Geometry: final body of the model. Coordinates: model frame, mm. Give positions to 0.01 mm unless a question says otherwise; leave off trailing zeros. Write each loop counter-clockwise with the first axis right and the second up, starting at its lowest first coordinate (ties: lowest second). Pieces come first, ordered by that corner, then holes.
```python
from build123d import *

# Parameters (mm, degrees)
SKETCH1_W           = 431.8
SKETCH1_H           = 381
BOSS_EXTRUDE1_DEPTH = 3.175
SKETCH7_R           = 14.3129
SKETCH7_R_2         = 2.5527
AXLE_HOLES_DEPTH    = 288.946419712
SKETCH10_R          = 3.2385
CUT_EXTRUDE5_DEPTH  = 288.946419712
CUT_EXTRUDE4_START  = -3.175
CUT_EXTRUDE4_DEPTH  = 3.175


# Read off the part's stored shape, not the designer's step: Cut-Extrude4
with BuildPart() as part:
    # Sketch1 → Boss-Extrude1 (new body)
    with BuildSketch(Plane(origin=(0, 0, 0), x_dir=(1, 0, 0), z_dir=(0, 1, 0))):
        Rectangle(SKETCH1_W, SKETCH1_H)
    extrude(amount=BOSS_EXTRUDE1_DEPTH)

    # Sketch7 → Axle Holes (cut, through all)
    with BuildSketch(Plane(origin=(0, 3.175, 0), x_dir=(1, 0, 0), z_dir=(0, 1, 0))):
        with Locations(Location((124.4092, -152.4, 0), (0, 0, 270))):
            Circle(SKETCH7_R)
        with Locations(Location((124.4092, 152.4, 0), (0, 0, 270))):
            Circle(SKETCH7_R)
        with Locations(Location((25.4, 152.4, 0), (0, 0, 270))):
            Circle(SKETCH7_R)
        with Locations(Location((25.4, -152.4, 0), (0, 0, 270))):
            Circle(SKETCH7_R)
        with Locations(Location((0, 152.4, 0), (0, 0, 270))):
            Circle(SKETCH7_R_2)
        with Locations(Location((7.439487758, 170.360512242, 0), (0, 0, 270))):
            Circle(SKETCH7_R_2)
        with Locations(Location((25.4, 177.8, 0), (0, 0, 270))):
            Circle(SKETCH7_R_2)
        with Locations(Location((43.360512242, 170.360512242, 0), (0, 0, 270))):
            Circle(SKETCH7_R_2)
        with Locations(Location((25.4, -127, 0), (0, 0, 270))):
            Circle(SKETCH7_R_2)
        with Locations(Location((43.360512242, -134.439487758, 0), (0, 0, 270))):
            Circle(SKETCH7_R_2)
        with Locations(Location((50.8, -152.4, 0), (0, 0, 270))):
            Circle(SKETCH7_R_2)
        with Locations(Location((43.360512242, -170.360512242, 0), (0, 0, 270))):
            Circle(SKETCH7_R_2)
        with Locations(Location((50.8, 152.4, 0), (0, 0, 270))):
            Circle(SKETCH7_R_2)
        with Locations(Location((43.360512242, 134.439487758, 0), (0, 0, 270))):
            Circle(SKETCH7_R_2)
        with Locations(Location((25.4, 127, 0), (0, 0, 270))):
            Circle(SKETCH7_R_2)
        with Locations(Location((7.439487758, 134.439487758, 0), (0, 0, 270))):
            Circle(SKETCH7_R_2)
        with Locations(Location((25.4, -177.8, 0), (0, 0, 270))):
            Circle(SKETCH7_R_2)
        with Locations(Location((7.439487758, -170.360512242, 0), (0, 0, 270))):
            Circle(SKETCH7_R_2)
        with Locations(Location((0, -152.4, 0), (0, 0, 270))):
            Circle(SKETCH7_R_2)
        with Locations(Location((7.439487758, -134.439487758, 0), (0, 0, 270))):
            Circle(SKETCH7_R_2)
    extrude(amount=-AXLE_HOLES_DEPTH, mode=Mode.SUBTRACT)

    # Sketch10 → Cut-Extrude5 (cut, through all)
    with BuildSketch(Plane(origin=(0, 3.175, 0), x_dir=(1, 0, 0), z_dir=(0, 1, 0))):
        with Locations(Location((-9.525, -182.394929259, 0), (0, 0, 270))):
            Circle(SKETCH10_R)
        with Locations(Location((74.9046, -184.15, 0), (0, 0, 270))):
            Circle(SKETCH10_R)
        with Locations(Location((74.9046, -133.35, 0), (0, 0, 270))):
            Circle(SKETCH10_R)
        with Locations(Location((167.623037844, -168.275, 0), (0, 0, 270))):
            Circle(SKETCH10_R)
        with Locations(Location((167.623037844, 168.275, 0), (0, 0, 90))):
            Circle(SKETCH10_R)
        with Locations(Location((74.9046, 184.15, 0), (0, 0, 90))):
            Circle(SKETCH10_R)
        with Locations(Location((74.9046, 133.35, 0), (0, 0, 90))):
            Circle(SKETCH10_R)
        with Locations(Location((-9.525, 182.394929259, 0), (0, 0, 90))):
            Circle(SKETCH10_R)
    extrude(amount=-CUT_EXTRUDE5_DEPTH, mode=Mode.SUBTRACT)

    # Cut-Extrude4 outline → Cut-Extrude4 (cut)
    with BuildSketch(Plane(origin=(0, 3.175, 0), x_dir=(1, 0, 0), z_dir=(0, 1, 0)).offset(CUT_EXTRUDE4_START)):
        with BuildLine():
            Line((170.541801783, -180.70028669), (133.121928175, -189.490408029))
            ThreePointArc((133.121928175, -189.490408029), (128.794713317, -190.246760402), (124.4092, -190.5))
            Line((124.4092, -190.5), (215.9, -190.5))
            Line((215.9, -190.5), (215.9, 190.5))
            Line((215.9, 190.5), (124.4092, 190.5))
            ThreePointArc((124.4092, 190.5), (128.794713317, 190.246760402), (133.121928175, 189.490408029))
            Line((133.121928175, 189.490408029), (170.541801783, 180.70028669))
            ThreePointArc((170.541801783, 180.70028669), (179.603701854, 172.676206897), (177.891266843, 160.694076212))
            Line((177.891266843, 160.694076212), (155.060629846, 129.770376751))
            ThreePointArc((155.060629846, 129.770376751), (112.346540244, 0), (155.060629846, -129.770376751))
            Line((155.060629846, -129.770376751), (177.891266843, -160.694076212))
            ThreePointArc((177.891266843, -160.694076212), (179.603701854, -172.676206897), (170.541801783, -180.70028669))
        make_face()
    extrude(amount=CUT_EXTRUDE4_DEPTH, mode=Mode.SUBTRACT)


solid = part.part
```
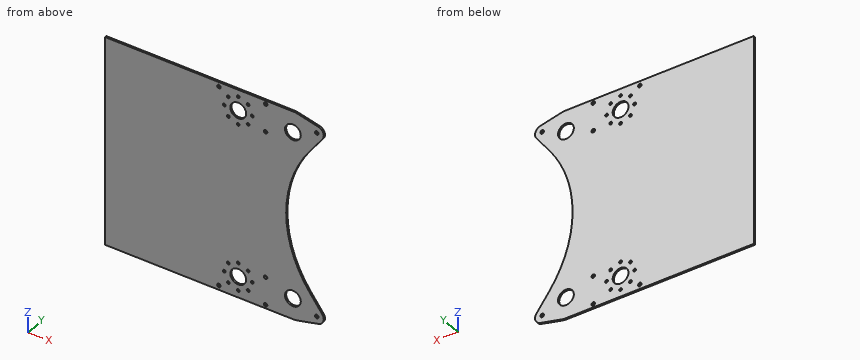
Item 1: Pin query (flat end, axial travel): pin 1 Ø4.5 at (x, z) = (25.4, 127) entering from +Y. Return the tip coordinate at first contact, or that it passes through.
Found:
pin 1: passes through
Item 2: Line query: L1, parallel to Z at x = 53, y = 2.45; L2, parallel to X at y = 2.8, z = 133; L3, parallel to X at y = 0.65, z = -151. Output: solid intervals per line, ascending.
Found:
L1: z = -190.5 to -153.69, -151.11 to 151.11, 153.69 to 190.5
L2: x = -215.9 to 5.33, 9.55 to 41.25, 45.47 to 71.69, 78.12 to 157.45
L3: x = -215.9 to -2.13, 2.13 to 11.16, 39.64 to 48.67, 52.93 to 110.16, 138.65 to 170.73
Item 3: Section C-C, the plane z = -33.5. Return the cut outline in (x, y) (3 decimals).
Found:
outline: (-215.9, 0) - (114.93, 0) - (114.93, 3.175) - (-215.9, 3.175) - close
Item 4: Section A-A, the plane z = -89. Return the cut outline in (x, y) (3 decimals).
Found:
outline: (-215.9, 0) - (131.295, 0) - (131.295, 3.175) - (-215.9, 3.175) - close
Item 5: Section B-B, the plane y = 0.9. State how many separate pieces and enclosed holes the cut face has, plus the area to 3 significant figures.
Found:
separate pieces: 1
enclosed holes: 28
area: 132,000 mm2
